Read the model definition and answer for the solid it produces. Units are mm, in the model's axes. A direction names the side the tool comes from. Coordinates: 2 decimals unless noted, no trailing zeros. Loops run counter-clockwise (first coordinate to the right, second up) from the corner with the lowest first, then second, coordinate; pieces in that order, holes last.
from build123d import *

# Parameters (mm, degrees)
F0_W     = 10
F0_H     = 6
F1_DEPTH = 200


with BuildPart() as f1:
    # F0 (on Right) → F1 (new body)
    with BuildSketch(Plane.YZ):
        with BuildLine():
            Line((-76, 0), (-70, 0))
            ThreePointArc((-70, 0), (-52.426407, 42.426407), (-10, 60))
            Line((-10, 60), (-10, 66))
            ThreePointArc((-10, 66), (-56.669048, 46.669048), (-76, 0))
        make_face()
        with Locations((-5, 63)):
            Rectangle(F0_W, F0_H)
    extrude(amount=F1_DEPTH)


solid = f1.part
Item 1: A cutting plane is placed at A-A on x = 154.5. Determine the outline of the cut face in (y, z), then the cut area to 3 significant figures.
Numbers:
outline: (-76, 0) - (-70, 0) arc R60 cw to (-10, 60) - (0, 60) - (0, 66) - (-10, 66) arc R66 ccw to start
area: 654 mm2
Item 2: A cutting plane is placed at B-B on y = -54. Determine the outline of the cut face in (x, z), then the cut area to 3 significant figures.
Numbers:
outline: (0, 40.79) - (200, 40.79) - (200, 49.19) - (0, 49.19) - close
area: 1,680 mm2
Item 3: Find the intervals of material crossed by line 1 along Y through (x, z) = (142.5, 11); line 2 along Z through (x, y) = (168, -12); line 3 along Y through (x, z) = (182.5, 52.5), in increasing order.
Numbers:
line 1: y = -75.08 to -68.98
line 2: z = 59.97 to 65.97
line 3: y = -50 to -39.05
Item 4: A cutting plane is placed at C-C on z = 49.5. Determine the outline of the cut face in (x, y).
Numbers:
outline: (0, -53.65) - (200, -53.65) - (200, -43.91) - (0, -43.91) - close
Item 5: Which of the six approach directions +Z, -Z, +X, -X, +Y, -Y give full straight-line access (tool end or side, diameter ignored) to faces 1 (the face through (99, -5, 66)), 2 (the face through (99, -5, 60))?
Numbers:
face 1: +Z, +X, -X, +Y, -Y
face 2: -Z, +X, -X, +Y
Item 6: Given pin 1 (3 mm diameter, centred on x = 72, y = -6, fed in from -Z); pin 2 (12 mm diameter, centred on x = 177, y = -38, fed in from -Z); pin 3 (5 mm diameter, centred on x = 40.5, z = 29.5, fed in from -Y); pin 4 (8 mm diameter, centred on y = -52.5, z = 51.5, fed in from +X), each flat-ended and moving along its own axis, determine where each tip first touches the part or whether it passes through.
Numbers:
pin 1: stops at z = 60
pin 2: stops at z = 49.44
pin 3: stops at y = -70.22
pin 4: stops at x = 200
